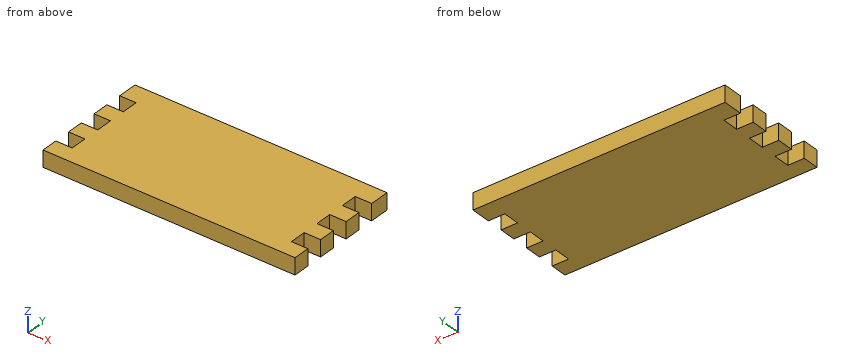
```python
from build123d import *

# Parameters (mm, degrees)
F0_W     = 10
F0_H     = 10
F1_DEPTH = 10


# Not quite as in the source:
# - a feature names something its author has since deleted; it is built from what else it names


with BuildPart() as f1:
    # F0 (on Top) → F1 (new body)
    with BuildSketch(Plane.XY):
        Polygon((-2.2346749902, 36.9413525529), (-135.6346749902, 36.9413525529), (-135.6346749902, 26.9413525529), (-135.6346749902, 16.9413525529), (-135.6346749902, 6.9413525529), (-135.6346749902, -3.0586474471), (-135.6346749902, -13.0586474471), (-135.6346749902, -23.0586474471), (-135.6346749902, -33.0586474471), (-2.2346749902, -33.0586474471), (-2.2346749902, -23.0586474471), (-2.2346749902, -13.0586474471), (-2.2346749902, -3.0586474471), (-2.2346749902, 6.9413525529), (-2.2346749902, 16.9413525529), (-2.2346749902, 26.9413525529), align=None)
        with Locations((-140.6346749902, 31.9413525529)):
            Rectangle(F0_W, F0_H)
        with Locations((-140.6346749902, 11.9413525529)):
            Rectangle(F0_W, F0_H)
        with Locations((-140.6346749902, -8.0586474471)):
            Rectangle(F0_W, F0_H)
        with Locations((-140.6346749902, -28.0586474471)):
            Rectangle(F0_W, F0_H)
        with Locations((2.7653250098, 31.9413525529)):
            Rectangle(F0_W, F0_H)
        with Locations((2.7653250098, 11.9413525529)):
            Rectangle(F0_W, F0_H)
        with Locations((2.7653250098, -8.0586474471)):
            Rectangle(F0_W, F0_H)
        with Locations((2.7653250098, -28.0586474471)):
            Rectangle(F0_W, F0_H)
        Polygon((-145.6346749902, 38.9413525529), (-145.6346749902, 36.9413525529), (-135.6346749902, 36.9413525529), (-2.2346749902, 36.9413525529), (7.7653250098, 36.9413525529), (7.7653250098, 38.9413525529), align=None)
    extrude(amount=F1_DEPTH)


solid = f1.part
```
Model file for the job. Use its own axes, mm. Coordinates: 2 decimals unless noted, no trailing zeros. Loops run counter-clockwise (first coordinate to the right, second up) from the corner with the lowest first, then second, coordinate; pieces in that order, holes last. Notation, with made-up numbers: (-34.5, 61) - (-18.5, 61) arc R13 cw to (-18.5, 75) - close; hole circle Ø4 at (-17, -0.5). An arc over 180 degrees is marked (long way). Answer as a JSON object with one key per item and string values. Group by question number.
(1) Cut at B-B (y = 19). Give the cut face in (x, z), then the cut area to 3 significant figures.
(2) Flat gauge pins, fed straight in: pin 1 (6 mm diameter, centred on y = 0.5, z = 5, fed in from -X); pin 2 (12 mm diameter, centred on x = -70, y = 31, fed in from -Z); pin 3 (5 mm diameter, centred on y = -18.5, z = 3.5, fed in from +X). Where does each tip first touch, or does it go through?
(3) Probe line 1 along Y through (x, z) = (0, 6); line 2 along X through (y, z) = (20.5, 4.5). List the from-to ranges inside material, lowest first.
(4) Cut at A-A (z = 5.5). Give the cut face in (x, y), then the cut area to 3 significant figures.
Geometry says:
{
 "1": {"outline": "(-135.63, 0) - (-2.23, 0) - (-2.23, 10) - (-135.63, 10) - close", "area": "1,330 mm^2"},
 "2": {"pin 1": "stops at x = -135.63", "pin 2": "stops at z = 0", "pin 3": "stops at x = -2.23"},
 "3": {"line 1": "y = -33.06 to -23.06, -13.06 to -3.06, 6.94 to 16.94, 26.94 to 38.94", "line 2": "x = -135.63 to -2.23"},
 "4": {"outline": "(-145.63, -33.06) - (7.77, -33.06) - (7.77, -23.06) - (-2.23, -23.06) - (-2.23, -13.06) - (7.77, -13.06) - (7.77, -3.06) - (-2.23, -3.06) - (-2.23, 6.94) - (7.77, 6.94) - (7.77, 16.94) - (-2.23, 16.94) - (-2.23, 26.94) - (7.77, 26.94) - (7.77, 38.94) - (-145.63, 38.94) - (-145.63, 26.94) - (-135.63, 26.94) - (-135.63, 16.94) - (-145.63, 16.94) - (-145.63, 6.94) - (-135.63, 6.94) - (-135.63, -3.06) - (-145.63, -3.06) - (-145.63, -13.06) - (-135.63, -13.06) - (-135.63, -23.06) - (-145.63, -23.06) - close", "area": "10,400 mm^2"}
}
